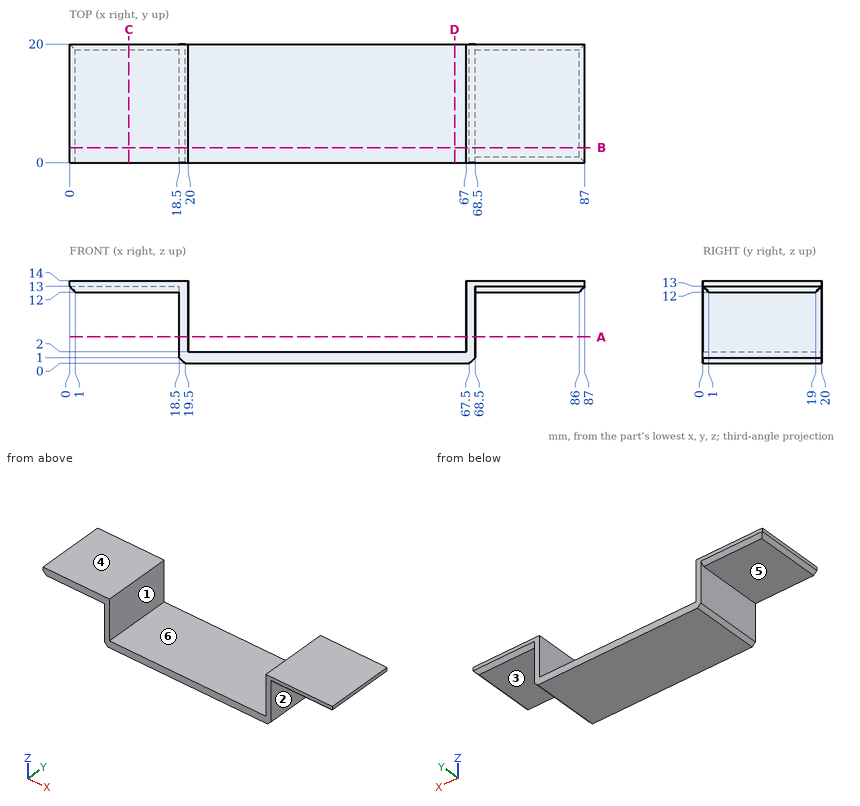
Check sheet for the drawn part. Datum: minimum x, y, z corner. Units: mm. A direction names the side the tool comes from. Give positions to 0.01 mm unless a question says otherwise; leave off trailing zeros. Order: outer loops, then holes, each group sorted by start corner. A loop starts at its lowest first (then second) coordinate and runs counter-clockwise, first axis right, second up. Notation, with made-up numbers: (-10.75, 13.25) - (15.25, 13.25) arc R8 ccw to (15.25, 20.25) - close; hole circle Ø10 at (-34, -37). An arc over 180 degrees is marked (long way). Write item = value, one per line. Start each with the question number.
1) Gauge pin test, flat ends, axial feed: pin 1 Ø1 at (y, z) = (9, 5) entering from -X; pin 2 Ø1.5 at (x, y) = (59.5, 7) entering from +Z. Record the tip position at first contact, or that the pin passes through.
2) Section check D-D (x = 65). Enter the section's corners in (y, z), then the cut area to 3 significant figures.
3) Scan lines: L1, parallel to X at y = 2, z = 13.5; L2, parallel to X at y = 6, z = 11.5; L3, parallel to Z at x = 66, y = 2.5. Record each from-to range of solid material in increasing order.
4) Access from +Z, -Z, +X, -X, +Y, -Y to the whole of each face (thin tool, end or side, straight path). Record for the marked faces 4, 5 and 6.
5) Section check B-B (y = 2.5). Enter the section's corners in (x, z), then the cut area to 3 significant figures.
6) Section check C-C (x = 10). Enter the section's corners in (y, z), then the cut area to 3 significant figures.
7) Draft check along X on the marked faces 1, 2 and 3. Enter one of: released by +X, released by -X, zero draft, split by the parting line, or undercut.
8) Section check A-A (z = 4.5). Enter the section's corners in (x, y), then the cut area to 3 significant figures.
Geometry check:
q1.pin_1 = 18.5
q1.pin_2 = 2
q2.outline = (0, 0) - (20, 0) - (20, 2) - (0, 2) - close
q2.area = 40.0 mm2
q3.L1 = 0 to 20, 67 to 87
q3.L2 = 18.5 to 20, 67 to 68.5
q3.L3 = 0 to 2
q4.face_4 = +Z, +X, -X, +Y, -Y
q4.face_5 = -Z, -X, +Y, -Y
q4.face_6 = +Z, +Y, -Y
q5.outline = (0, 13) - (1, 12) - (18.5, 12) - (18.5, 1) - (19.5, 0) - (67.5, 0) - (68.5, 1) - (68.5, 12) - (86, 12) - (87, 13) - (87, 14) - (67, 14) - (67, 2) - (20, 2) - (20, 14) - (0, 14) - close
q5.area = 208 mm2
q6.outline = (0, 12) - (19, 12) - (20, 13) - (20, 14) - (0, 14) - close
q6.area = 39.5 mm2
q7.face_1 = undercut
q7.face_2 = released by +X
q7.face_3 = zero draft
q8.outline = (18.5, 0) - (20, 0) - (20, 20) - (18.5, 20) - close; (67, 0) - (68.5, 0) - (68.5, 20) - (67, 20) - close
q8.area = 60.0 mm2
